The model under review builds one solid part; all positions refer to its coordinate system, in mm. Face numbers are marked on the shaded views. A direction names the side the tool comes from. Give positions to 0.01 mm unless a question says otherwise; leave off trailing zeros. Order: outer loops, then holes, each group sorted by start corner. A loop starts at its lowest first (then second) coordinate and runs counter-clockwise, first axis right, second up. Notation, with made-up numbers: (36, 85.5) - (46, 85.5) arc R31 ccw to (46, 123.5) - close; hole circle Ø5 at (-16.5, 24). An arc over 180 degrees is marked (long way). Use CSV: the item, a comma, the result in double quotes.
```python
from build123d import *

# Parameters (mm, degrees)
F1_DEPTH = 25
F2_R     = 2
F3_DEPTH = 15
F4_R     = 1.99999


# Not quite as in the source:
# - a fillet or chamfer is up to 0.001 mm smaller than in the source, because OpenCascade refuses the exact size


with BuildPart() as f1:
    # F0 (on Top) → F1 (new body)
    with BuildSketch(Plane.XY):
        Polygon((15, 0), (0, 0), (0, -15), (5, -15), (5, -5), (15, -5), align=None)
    extrude(amount=F1_DEPTH)

    # F2
    f2_edges = [f1.edges().sort_by_distance(p)[0] for p in [
        (5, -5, 12.5),
        (0, 0, 12.5),
    ]]
    fillet(f2_edges, radius=F2_R)

    # F0 (on Top) → F3 (join)
    with BuildSketch(Plane.XY):
        Polygon((5, -15), (0, -15), (0, -17), (7, -17), (7, -15), align=None)
        Polygon((17, 0), (15, 0), (15, -5), (15, -7), (17, -7), align=None)
    extrude(amount=F3_DEPTH)

    # F4 (radius 2 in the source; OpenCascade refuses exactly that, so slightly less here)
    f4_edges = [f1.edges().sort_by_distance(p)[0] for p in [
        (5, -15, 7.5),
        (15, -5, 7.5),
    ]]
    fillet(f4_edges, radius=F4_R)


solid = f1.part
```
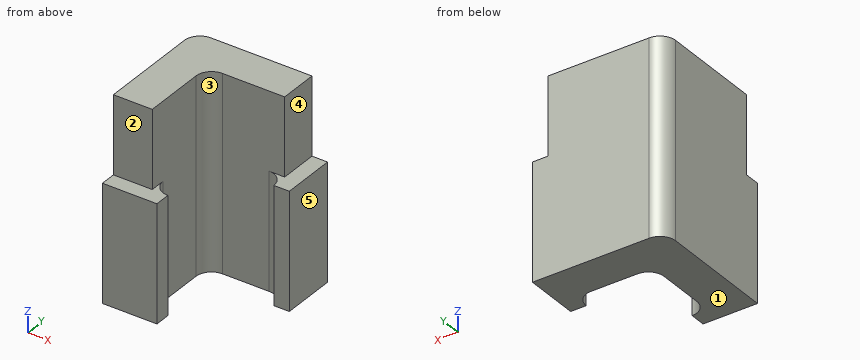
Item 1: Wall thickness on L1, parallel to X at y = -13.75, z = 18; L2, parallel to Y at x = 10.25, z = 4; L3, parallel to X at y = -6.5, z = 12.5: over which ranges is each line inside the solid? List them lowest first.
Results list:
L1,"x = 0 to 5"
L2,"y = -5 to 0"
L3,"x = 0 to 5.06, 14.94 to 17"
Item 2: Tool access review of the marked faces 4 and 5: name each direction out of +Z, -Z, +X, -X, +Y, -Y from which nothing blocks a thin tool from reaching the whole face with its end or side.
Results list:
face 4,"+Z, +X, +Y, -Y"
face 5,"+Z, -Z, +X, +Y, -Y"
Item 3: Clearance check with flat-ended pins moving along their axes: pin 1 (6.5 mm diameter, centred on x = 10.5, z = 12, fed in from -Y); pin 2 (0.6 mm diameter, centred on x = 16, z = 4.5, fed in from -Y); pin 3 (8 mm diameter, centred on x = 10, z = 21, fed in from -Y). State where each tip first meets the part, or that it passes through.
Results list:
pin 1,"stops at y = -5.15"
pin 2,"stops at y = -7"
pin 3,"stops at y = -5.27"
Item 4: Mouldability with a two-part tool opening along Y and no side actions: class the marked faces 1, 2 and 3 as pulls with the +Y half, pulls with the -Y half, needs draft (parallel to the pull), parting line crosses it, or undercut.
Results list:
face 1,"needs draft"
face 2,"pulls with the -Y half"
face 3,"undercut"
Item 5: Take a section at C-C, the plane x = 2.75. Give the boundary of the cut face in (y, z).
Results list:
outline,"(-17, 0) - (0, 0) - (0, 25) - (-15, 25) - (-15, 15) - (-17, 15) - close"
Item 6: Take a section at B-B, the plane x = 5.75. Give the boundary of the cut face in (y, z), and give its area (3 significant figures).
Results list:
outline,"(-17, 0) - (-14.56, 0) - (-14.56, 15) - (-17, 15) - close; (-5.44, 0) - (0, 0) - (0, 25) - (-5.44, 25) - close"
area,"173 mm2"
Item 7: Take a section at D-D, the plane y = -8. Give the boundary of the cut face in (x, z), and give its area (3 significant figures).
Results list:
outline,"(0, 0) - (5, 0) - (5, 25) - (0, 25) - close"
area,"125 mm2"
